Geometry check sheet. Reference: the model listing, model coordinates, mm. A direction names the side the tool comes from. Coordinates: 2 decimals unless noted, no trailing zeros. Write each loop counter-clockwise with the first axis right and the second up, starting at its lowest first coordinate (ties: lowest second). Pieces come first, ordered by that corner, then holes.
from build123d import *

# Parameters (mm, degrees)
SKETCH1_R           = 6
BOSS_EXTRUDE1_DEPTH = 25
SKETCH2_R           = 2.75
CUT_EXTRUDE1_DEPTH  = 33.5
SKETCH3_W           = 34
SKETCH3_H           = 34
SKETCH3_R           = 6
BOSS_EXTRUDE2_DEPTH = 5
SKETCH4_R           = 9
SKETCH4_R_2         = 6
BOSS_EXTRUDE3_DEPTH = 4


with BuildPart() as part:
    # Sketch1 → Boss-Extrude1 (new body)
    with BuildSketch(Plane(origin=(0, 0, 0), x_dir=(1, 0, 0), z_dir=(0, 1, 0))):
        Polygon((30, -21.5), (-30, -21.5), (-30, 11), (-17, 11), (-17, 21.5), (17, 21.5), (17, 11), (30, 11), align=None)
        with Locations((0, 3.5)):
            Circle(SKETCH1_R, mode=Mode.SUBTRACT)
    extrude(amount=BOSS_EXTRUDE1_DEPTH)

    # Sketch2 → Cut-Extrude1 (cut, through all)
    with BuildSketch(Plane(origin=(0, 0, -11), x_dir=(-1, 0, 0), z_dir=(0, 0, -1))):
        with Locations((-23, 19)):
            Circle(SKETCH2_R)
        with Locations((-23, 6)):
            Circle(SKETCH2_R)
        with Locations((23, 6)):
            Circle(SKETCH2_R)
        with Locations((23, 19)):
            Circle(SKETCH2_R)
    extrude(amount=-CUT_EXTRUDE1_DEPTH, mode=Mode.SUBTRACT)

    # Sketch3 → Boss-Extrude2 (add)
    with BuildSketch(Plane(origin=(0, 25, 0), x_dir=(1, 0, 0), z_dir=(0, 1, 0))):
        with Locations((0, 4.5)):
            Rectangle(SKETCH3_W, SKETCH3_H)
        with Locations((0, 3.5)):
            Circle(SKETCH3_R, mode=Mode.SUBTRACT)
    extrude(amount=BOSS_EXTRUDE2_DEPTH)

    # Sketch4 → Boss-Extrude3 (add)
    with BuildSketch(Plane(origin=(0, 30, 0), x_dir=(1, 0, 0), z_dir=(0, 1, 0))):
        with Locations((0, 3.5)):
            Circle(SKETCH4_R)
        with Locations((0, 3.5)):
            Circle(SKETCH4_R_2, mode=Mode.SUBTRACT)
    extrude(amount=BOSS_EXTRUDE3_DEPTH)


solid = part.part
1. Access from +Z, -Z, +X, -X, +Y, -Y to the whole of each face (thin tool, end or side, straight path). Record for faces 1 (the flat face through (23, 12, -11)), 2 (the flat face through (0, 12, 21.5)), 3 (the flat face through (-24, 12, -11)), 4 (the flat face through (0, 27, 12.5)).
Computed values:
face 1: -Z, +X, +Y, -Y
face 2: +Z, +X, -X, +Y, -Y
face 3: -Z, -X, +Y, -Y
face 4: +Z, +X, -X, +Y
2. Gauge pin test, flat ends, axial feed: pin 1 Ø4 at (x, y) = (1, 28) entering from +Z; pin 2 Ø6.5 at (x, y) = (22.5, 16) entering from -Z; pin 3 Ø1.5 at (y, z) = (28.5, 12) entering from -X; pin 4 Ø4.5 at (x, y) = (23, 19) entering from -Z. Record the tip position at first contact, or that the pin passes through.
Computed values:
pin 1: stops at z = 12.5
pin 2: stops at z = -11
pin 3: stops at x = -17
pin 4: passes through
3. Sectioned sample at D-D, the plane x = 0. Record the boundary of the cut face in (y, z), and give its area (3 significant figures).
Computed values:
outline: (0, -21.5) - (30, -21.5) - (30, -12.5) - (34, -12.5) - (34, -9.5) - (0, -9.5) - close; (0, 2.5) - (34, 2.5) - (34, 5.5) - (30, 5.5) - (30, 12.5) - (25, 12.5) - (25, 21.5) - (0, 21.5) - close
area: 909 mm2
4. Sectioned sample at B-B, the plane z = -3.5. Record the boundary of the cut face in (x, y), and give its area (3 significant figures).
Computed values:
outline: (-30, 0) - (-6, 0) - (-6, 34) - (-9, 34) - (-9, 30) - (-17, 30) - (-17, 25) - (-30, 25) - close; (6, 0) - (30, 0) - (30, 25) - (17, 25) - (17, 30) - (9, 30) - (9, 34) - (6, 34) - close; hole circle Ø5.5 at (-23, 6); hole circle Ø5.5 at (-23, 19); hole circle Ø5.5 at (23, 6); hole circle Ø5.5 at (23, 19)
area: 1,240 mm2
5. Sectioned sample at C-C, the plane x = -23. Record the boundary of the cut face in (y, z), and give its area (3 significant figures).
Computed values:
outline: (0, -11) - (3.25, -11) - (3.25, 21.5) - (0, 21.5) - close; (8.75, -11) - (16.25, -11) - (16.25, 21.5) - (8.75, 21.5) - close; (21.75, -11) - (25, -11) - (25, 21.5) - (21.75, 21.5) - close
area: 455 mm2
6. Thickness scan on line 1 along Y through (x, z) = (23, 6); line 2 along Z through (x, y) = (0, 2.5); line 3 along X through (y, z) = (21, 6.5). Record the ranges inside material, lowest first.
Computed values:
line 1: y = 0 to 3.25, 8.75 to 16.25, 21.75 to 25
line 2: z = -21.5 to -9.5, 2.5 to 21.5
line 3: x = -30 to -24.89, -21.11 to 21.11, 24.89 to 30
7. Sectioned sample at A-A, the plane y = 19. Record the boundary of the cut face in (x, z), and give its area (3 significant figures).
Computed values:
outline: (-30, -11) - (-25.75, -11) - (-25.75, 21.5) - (-30, 21.5) - close; (-20.25, -11) - (-17, -11) - (-17, -21.5) - (17, -21.5) - (17, -11) - (20.25, -11) - (20.25, 21.5) - (-20.25, 21.5) - close; (25.75, -11) - (30, -11) - (30, 21.5) - (25.75, 21.5) - close; hole circle Ø12 at (0, -3.5)
area: 1,840 mm2
8. Draft check along Y on faces 5 (the flat face through (0, 0, 4)), 6 (the cylindrical face through (-7.14, 31.97, 1.98)), 7 (the cylindrical face through (-20.253, 19.121, 5.023)). Enter one of: released by +Y, released by -Y, zero draft, split by the parting line, or undercut.
Computed values:
face 5: released by -Y
face 6: zero draft
face 7: undercut
